Model file for the job. Use its own axes, mm. A direction names the side the tool comes from. Round coordinates to 2 decimals unless told otherwise and drop trailing zeros. Loops run counter-clockwise (first coordinate to the right, second up) from the corner with the lowest first, then second, coordinate; pieces in that order, holes last. Notation, with made-up numbers: M 67.25,-28 L 83.25,-28 A28 cw 83.25,-10 Z; hole C 1,55.5 d7. An arc over 180 degrees is marked long. Answer in a Markdown table with one row per item.
from build123d import *

# Parameters (mm, degrees)
SKETCH1_R           = 2.5
BOSS_EXTRUDE1_DEPTH = 3
BOSS_EXTRUDE2_DEPTH = 15
BOSS_EXTRUDE2_DRAFT = 4
FILLET2_R           = 1
FILLET3_R           = 1
FILLET4_R           = 1
FILLET5_R           = 1
FILLET6_R           = 1
FILLET7_R           = 1


with BuildPart() as part:
    # Sketch1 → Boss-Extrude1 (new body)
    with BuildSketch(Plane(origin=(0, 0, 0), x_dir=(1, 0, 0), z_dir=(0, 1, 0))):
        Polygon((0, 0), (-25.5, 0), (-25.5, -19.76), (-20, -19.76), (-20, -6), (0, -6), align=None)
        with Locations(Location((-7.5, -3, 0), (0, 0, 270))):
            Circle(SKETCH1_R, mode=Mode.SUBTRACT)
        with Locations(Location((-22.5, -3, 0), (0, 0, 270))):
            Circle(SKETCH1_R, mode=Mode.SUBTRACT)
    extrude(amount=BOSS_EXTRUDE1_DEPTH)


with BuildPart() as boss_extrude2_tool:
    # Sketch3 → Boss-Extrude2 (with draft: the straight prism first)
    with BuildSketch(Plane(origin=(0, 3, 0), x_dir=(1, 0, 0), z_dir=(0, 1, 0))):
        with BuildLine():
            ThreePointArc((-20, -8.76), (-25.5, -14.26), (-20, -19.76))
            Line((-20, -19.76), (-20, -8.76))
        make_face()
    extrude(amount=BOSS_EXTRUDE2_DEPTH)
    # Boss-Extrude2: the draft: its side faces are tilted about the plane it starts from
    boss_extrude2_sides = [boss_extrude2_tool.faces().sort_by_distance(p)[0] for p in [
        (-25.5, 10.5, 14.26),
        (-20, 10.5, 14.26),
    ]]
    draft(boss_extrude2_sides, Plane(origin=(0, 3, 0), x_dir=(1, 0, 0), z_dir=(0, 1, 0)), BOSS_EXTRUDE2_DRAFT)


with BuildPart() as part_1:
    add(part.part)

    # Boss-Extrude2: add boss_extrude2_tool
    add(boss_extrude2_tool.part)

    # Fillet2
    fillet2_edges = [part_1.edges().sort_by_distance(p)[0] for p in [
        (-20, 1.5, 6),
    ]]
    fillet(fillet2_edges, radius=FILLET2_R)

    # Fillet3
    # the kernel refuses this fillet: 1 mm, written as the material it takes off along each edge
    with BuildSketch(Plane(origin=(-20, -6, 19.76), x_dir=(0, 0, -1), z_dir=(0, 1, 0))) as fillet3_piece_1:
        with BuildLine():
            CenterArc((FILLET3_R, FILLET3_R), FILLET3_R, 180, 90)
            Line((0, FILLET3_R), (-FILLET3_R * 0.02, FILLET3_R))
            Line((-FILLET3_R * 0.02, FILLET3_R), (-FILLET3_R * 0.02, -FILLET3_R * 0.02))
            Line((-FILLET3_R * 0.02, -FILLET3_R * 0.02), (FILLET3_R, -FILLET3_R * 0.02))
            Line((FILLET3_R, -FILLET3_R * 0.02), (FILLET3_R, 0))
        make_face()
    extrude(amount=15, mode=Mode.SUBTRACT)

    # Fillet4
    fillet4_edges = [part_1.edges().sort_by_distance(p)[0] for p in [
        (-25.5, 1.5, 19.76),
    ]]
    fillet(fillet4_edges, radius=FILLET4_R)

    # Fillet5
    fillet5_edges = [part_1.edges().sort_by_distance(p)[0] for p in [
        (-25.5, 1.5, 0),
    ]]
    fillet(fillet5_edges, radius=FILLET5_R)

    # Fillet6
    fillet6_edges = [part_1.edges().sort_by_distance(p)[0] for p in [
        (0, 1.5, 0),
    ]]
    fillet(fillet6_edges, radius=FILLET6_R)

    # Fillet7
    fillet7_edges = [part_1.edges().sort_by_distance(p)[0] for p in [
        (0, 1.5, 6),
    ]]
    fillet(fillet7_edges, radius=FILLET7_R)


solid = part_1.part
1. Pin check, flat tips, straight feed: pin 1 (7 mm diameter, centred on x = -11.5, z = 5.5, fed in from +Y); pin 2 (1.5 mm diameter, centred on x = -8.5, y = 2, fed in from +Z); pin 3 (1 mm diameter, centred on y = 3, z = 12, fed in from +X). Stop position of each tip, or through.
Verdict:
| item | result |
|---|---|
| pin 1 | stops at y = 3 |
| pin 2 | stops at z = 6 |
| pin 3 | stops at x = -20 |
2. Mould opens along X. For faces 4 (the flat face through (-25.5, 1, 10)), 5 (the flat face through (-20, 1, 13)), 6 (the cylindrical face through (-20, 1, 3)), 7 (the flat face through (-13, 3, 4)) say: +X half, -X half, draft (parallel to the pull), parting line (faces both ways), or undercut.
Verdict:
| item | result |
|---|---|
| face 4 | -X half |
| face 5 | +X half |
| face 6 | undercut |
| face 7 | draft |
3. Wall check: probe 1 along X at (y, z) = (1.65, 3); probe 2 along X at (y, z) = (1.5, 14); probe 3 along Z at (x, y) = (-23.25, 1). Give the ranges that are in metal, low to high.
Verdict:
| item | result |
|---|---|
| probe 1 | x = -25.5 to -25, -20 to -10, -5 to 0 |
| probe 2 | x = -25.5 to -20 |
| probe 3 | z = 0 to 0.62, 5.38 to 19.76 |
4. Saw through at D-D (y = 6.75). Write the cut outline in (x, z).
Verdict:
| item | result |
|---|---|
| outline | M -20.31,19.49 A5.24 ccw -20.26,9.03 L -20.26,19.44 A1 ccw Z |
5. Saw through at B-B (z = 3). Write the cut outline in (x, y), and give its area (3 significant figures).
Verdict:
| item | result |
|---|---|
| outline | M -25.5,0 L -25,0 L -25,3 L -25.5,3 Z; M -20,0 L -10,0 L -10,3 L -20,3 Z; M -5,0 L 0,0 L 0,3 L -5,3 Z |
| area | 46.5 mm² |
6. Saw through at A-A (x = -7.5). Write the cut outline in (y, z), and give its area (3 significant figures).
Verdict:
| item | result |
|---|---|
| outline | M 0,0 L 3,0 L 3,0.5 L 0,0.5 Z; M 0,5.5 L 3,5.5 L 3,6 L 0,6 Z |
| area | 3.00 mm² |
7. Tool access for faces 1 (the cylindrical face through (-25.215, 1.521, 19.459)), 2 (the flat face through (-10, 1, 6)), 3 (the flat face through (-24, 3, 19)): list every direction of +Z, -Z, +X, -X, +Y, -Y with a clear straight run to the whole face (end or side of a thin tool).
Verdict:
| item | result |
|---|---|
| face 1 | +Z, -X, +Y, -Y |
| face 2 | +Z, +X, +Y, -Y |
| face 3 | +Z, -X, +Y |
8. Saw through at C-C (x = -17.25). Write the cut outline in (y, z), and give its area (3 significant figures).
Verdict:
| item | result |
|---|---|
| outline | M 0,0 L 3,0 L 3,6 L 0,6 Z |
| area | 18.0 mm² |
